Verification items for the finished model (mm, model axes). A direction names the side the tool comes from. Coordinates: 2 decimals unless noted, no trailing zeros. Order: outer loops, then holes, each group sorted by start corner. A loop starts at its lowest first (then second) coordinate and runs counter-clockwise, first axis right, second up. Notation, with made-up numbers: (79, 81) -> (105, 81) arc R26 cw to (105, 96) -> close; hole circle Ø2 at (46, 32). An arc over 180 degrees is marked (long way). Write item = value, one per line. Start each with the question number.
1. Go/stop test with flat-tipped pins: P1, Ø0.9, axis at y = 4.5, z = 4, coming from the -X side; P2, Ø3, axis at y = -5.5, z = 5.5, coming from the -X side; P3, Ø3, axis at x = 3, z = 4, coming from the -Y side. Record where each tip stops, or that it passes through.
2. Cross-section at B-B on y = 0. Record the cut outline in (x, z).
3. Cross-section at A-A on x = 0. Record the cut outline in (y, z).
4. Cross-section at D-D on y = 6. Record the cut outline in (x, z).
5. Thickness scan on line 1 along Y through (x, z) = (0, 5.5); line 2 along Y through (x, z) = (1.5, 7.5); line 3 along X through (y, z) = (2.5, 8.5). Record the ranges inside material, lowest first. Write a range as from..to.
6. Set-up check for faces 1 (the flat face through (2, -4, 0)), 2 (the flat face through (0, 5, 5)): record each of +Z, -Z, +X, -X, +Y, -Y from which the full face is reachable in a straight line by a thin tool's end or side.
7. Cross-section at C-C on z = 5.25. Record the cut outline in (x, y).
from build123d import *

# Parameters (mm, degrees)
SKETCH_1_R      = 9
EXTRUDE_1_DEPTH = 10


with BuildPart() as part:
    # ｽｹｯﾁ1 → ﾎﾞｽ - 押し出し1 (new body)
    with BuildSketch(Plane.XY):
        Circle(SKETCH_1_R)
        with BuildLine():
            Line((-1, 5), (-1, 3.872983346))
            ThreePointArc((-1, 3.872983346), (0, -4), (1, 3.872983346))
            Line((1, 3.872983346), (1, 5))
            Line((1, 5), (-1, 5))
        make_face(mode=Mode.SUBTRACT)
    extrude(amount=EXTRUDE_1_DEPTH)


solid = part.part
Worked out:
q1.P1 = -8.04
q1.P2 = -8.06
q1.P3 = -8.87
q2.outline = (-9, 0) -> (-4, 0) -> (-4, 10) -> (-9, 10) -> close; (4, 0) -> (9, 0) -> (9, 10) -> (4, 10) -> close
q3.outline = (-9, 0) -> (-4, 0) -> (-4, 10) -> (-9, 10) -> close; (5, 0) -> (9, 0) -> (9, 10) -> (5, 10) -> close
q4.outline = (-6.71, 0) -> (6.71, 0) -> (6.71, 10) -> (-6.71, 10) -> close
q5.line_1 = -9..-4, 5..9
q5.line_2 = -8.87..-3.71, 3.71..8.87
q5.line_3 = -8.65..-3.12, 3.12..8.65
q6.face_1 = -Z, +X, -X, +Y, -Y
q6.face_2 = +Z, -Z
q7.outline = circle Ø18 at (0, 0); hole (-1, 3.87) arc R4 ccw (long way) to (1, 3.87) -> (1, 5) -> (-1, 5) -> close
